Input: part model. Units: mm. Frame: model coordinates. A direction names the side the tool comes from. Give positions to 0.01 mm unless a question says otherwise; leave off trailing zeros. Loops run counter-clockwise (first coordinate to the right, second up) from the corner with the lowest first, then second, coordinate; pieces in that order, holes last. Notation, with made-up numbers: M 52,37.25 L 70,37.25 A22 cw 70,62.25 Z; hole C -13,63 d10. An arc over 180 degrees is marked long. Answer as a JSON object with one key per item and string values. Group by question number.
1) Draft query along X for faces 4 (the flat face through (1, 0, 1)), 5 (the cylindrical face through (8.123, 56.439, 50.54)), 6 (the flat face through (-3, 6.35, 13)). Return one class per face: +X half, -X half, draft (parallel to the pull), parting line (faces both ways), or undercut.
2) Section query C-C on y = 117. Return loops of the section in (x, z).
3) Access query for faces 1 (the cylindrical face through (-2.75, 75.22, -12.4)), 2 (the cylindrical face through (-50.247, 56.439, 0.152)), 3 (the flat face through (0, 146.05, 0)). Directions: +Z, -Z, +X, -X, +Y, -Y. A direction counts if a zero-diameter tool reaches every point of the face in a straight line with its end or side. Return the directions, or none.
4) Section query D-D on x = -43.5. Return loops of the section in (y, z).
5) Section query B-B on x = 42. Return loops of the section in (y, z).
6) Ray query, L1, parallel to Z at x = 0, y = 75 (3 decimals); L2, parallel to Y at x = -12, z = 2; L3, parallel to Y at x = 24.5, z = -37.5. Return the intervals inside material, ascending.
7) First-contact query: P1, Ø8, axis at x = -8.5, y = 97, coming from the +Z side; P2, Ø5, axis at y = 27.5, z = -23, coming from the +X side; P3, Ø12, axis at x = -34.5, y = 24.5, coming from the +Z side. Flat tips, straight axial feed; report the tip coordinate or a pass-through.
Autodesk Inventor part; units mm, degrees
ref_plane "YZ Plane" through (0, 0, 0) normal (1, 0, 0) x (0, 1, 0)
ref_plane "XZ Plane" through (0, 0, 0) normal (0, 1, 0) x (-1, 0, 0)
ref_plane "XY Plane" through (0, 0, 0) normal (0, 0, 1) x (1, 0, 0)
sketch "Sketch1" plane through (0, 0, 0) normal (0, 1, 0) x (-1, 0, 0)
  circle A0 centre (0, 0) radius 53.975
  dimension "d0" = 107.95
extrude "Extrusion1" add sketch "Sketch1" along normal blind 107.95
sketch "Sketch2" plane through (0, 107.95, 0) normal (0, 1, 0) x (1, 0, 0)
  arc A0 (-1.614, -49.186) -> (-49.186, -1.614) centre (0, 0) ccw
  circle A1 centre (0, 0) radius 53.975
  line L0 (9.8864, -53.0619) -> (14.2923, -39.9886)
  line L1 (14.2923, -39.9886) -> (-59.1143, -15.2492)
  line L2 (-59.1143, -15.2492) -> (-53.975, 0)
  line L3 (-53.975, 0) -> (-49.186, -1.614)
  line L4 (-1.614, -49.186) -> (9.8864, -53.0619)
  dimension "d3" = 98.425
extrude "Extrusion2" cut sketch "Sketch2" against normal blind 101.6 contours L4 A1 L1 L0 A0 | L0 L1 A1 L3 A0
sketch "Sketch3" plane through (0, 6.35, 0) normal (0, 1, 0) x (1, 0, 0)
  circle A0 centre (0, 0) radius 12.7
  dimension "d7" = 25.4
extrude "Extrusion3" add sketch "Sketch3" along normal blind 139.7
ref_plane "Work Plane1" through (0, 6.35, 0) normal (0.9831, 0, -0.1832) x (0, 1, 0)
sketch "Sketch4" plane through (0, 6.35, 0) normal (0.9831, 0, -0.1832) x (0, 1, 0)
  circle A0 centre (120.65, 0) radius 3.175
  line L0 (139.7, -12.7) -> (139.7, 12.7)
  point P0 (-6.35, 0)
  dimension "d10" = 6.35
  dimension "d11" = 19.05
extrude "Extrusion4" cut sketch "Sketch4" along normal through all
sketch "Sketch5" plane through (0, 6.35, 0) normal (0.9831, 0, -0.1832) x (0, 1, 0)
  circle A0 centre (120.65, 0) radius 3.175
  circle A1 centre (120.65, 0) radius 3.175
  point P0 (-6.35, 0)
extrude "Extrusion5" cut sketch "Sketch5" against normal blind 139.7
fillet "Fillet2" radius 2.54 2 edges at (-49.186, 57.15, 1.614) (-1.614, 57.15, 49.186)
properties part number "Hand Holder"
Output:
{
 "1": {"face 4": "draft", "face 5": "-X half", "face 6": "undercut"},
 "2": {"outline": "C 0,0 d25.4"},
 "3": {"face 1": "+Y", "face 2": "+Z, +Y", "face 3": "+Z, -Z, +X, -X, +Y"},
 "4": {"outline": "M 0,-31.95 L 107.95,-31.95 L 107.95,-23.01 L 6.35,-23.01 L 6.35,31.95 L 0,31.95 Z"},
 "5": {"outline": "M 0,-33.9 L 107.95,-33.9 L 107.95,-25.65 L 6.35,-25.65 L 6.35,25.65 L 107.95,25.65 L 107.95,33.9 L 0,33.9 Z"},
 "6": {"L1": "z = -53.975 to -49.212, -12.7 to 12.7", "L2": "y = 0 to 123.83, 130.17 to 146.05", "L3": "y = 0 to 6.35"},
 "7": {"P1": "stops at z = 11.88", "P2": "stops at x = 49.93", "P3": "stops at z = -27.96"}
}
